Check sheet for the modelled part. Datum: model origin and axes. Units: mm. Face numbers are marked on the shaded views. A direction names the side the tool comes from. Round coordinates to 2 decimals unless told otherwise and drop trailing zeros. Write each loop counter-clockwise with the first axis right and the second up, starting at its lowest first coordinate (ties: lowest second). Pieces come first, ordered by that corner, then holes. Notation, with made-up numbers: M 41,33 L 93,33 A19 cw 93,49 Z; hole C 31,83 d2. An arc over 180 degrees is marked long. Answer in a Markdown table with one row per item.
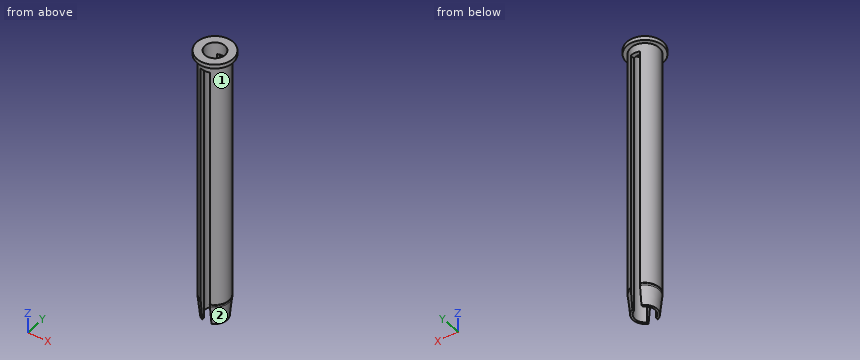
```python
from build123d import *

# Parameters (mm, degrees)
CHAFL_N2_SIZE           = 10
CHAFL_N2_SIZE2          = 1
REDONDEO1_R             = 10
SALIENTE_EXTRUIR1_START = -10.5
CROQUIS3_R              = 7.05
CROQUIS3_R_2            = 6.95
SALIENTE_EXTRUIR1_DEPTH = 0.2
CROQUIS2_W              = 4.5
CROQUIS2_H              = 17.325126262
CORTAR_EXTRUIR1_DEPTH   = 131
CHAFL_N3_SIZE           = 0.1
REDONDEO2_R             = 0.05


# Some blends are built 0.0001 mm under size
with BuildPart() as part:
    # Croquis1 → Revolución1 (revolve)
    with BuildSketch(Plane.YZ, mode=Mode.PRIVATE) as revoluci_n1_sk:
        Polygon((4.95, -68.5), (4.95, 68.5), (8.95, 68.5), (8.95, 66.5), (6.95, 66.5), (6.95, -68.5), align=None)
    revolve(revoluci_n1_sk.sketch.rotate(Axis((0, 0, 0), (0, 0, 1)), 90), axis=Axis((0, 0, 0), (0, 0, 1)))

    # Chaflán2
    chafl_n2_edges = [part.edges().sort_by_distance(p)[0] for p in [
        (6.95, 0, -68.5),
    ]]
    chafl_n2_side = [part.faces().sort_by_distance(p)[0] for p in [
        (6.95, 0, -1),
    ]]
    chamfer(chafl_n2_edges, length=CHAFL_N2_SIZE, length2=CHAFL_N2_SIZE2, reference=chafl_n2_side[0])

    # Redondeo1
    # the kernel refuses this fillet: 10 mm, written as the material it takes off along each edge
    with BuildSketch(Plane(origin=(0, 0, -58.5), x_dir=(-1, 0, 0), z_dir=(0, 1, 0))) as redondeo1_piece_1:
        with BuildLine():
            CenterArc((6.95 - REDONDEO1_R, REDONDEO1_R * 0.0498756211209), REDONDEO1_R, 354.289406863, 5.710593137)
            Line((6.95 - REDONDEO1_R * 0.00496280979001, -REDONDEO1_R * 0.0496280979001), (6.95, 0))
            Line((6.95, 0), (6.95, REDONDEO1_R * 0.0498756211209))
        make_face()
    revolve(axis=Axis((0, 0, -58.5), (0, 0, 1)), mode=Mode.SUBTRACT)

    # Croquis3 → Saliente-Extruir1 (add)
    with BuildSketch(Plane(origin=(0, 0, -68.5), x_dir=(1, 0, 0), z_dir=(0, 0, -1)).offset(SALIENTE_EXTRUIR1_START)):
        with Locations(Location((0, 0, 0), (0, 0, 180))):
            Circle(CROQUIS3_R)
        with Locations(Location((0, 0, 0), (0, 0, 180))):
            Circle(CROQUIS3_R_2, mode=Mode.SUBTRACT)
    extrude(amount=-SALIENTE_EXTRUIR1_DEPTH)

    # Croquis2 → Cortar-Extruir1 (cut)
    with BuildSketch(Plane(origin=(0, 0, -68.5), x_dir=(1, 0, 0), z_dir=(0, 0, -1))):
        Rectangle(CROQUIS2_W, CROQUIS2_H)
    extrude(amount=-CORTAR_EXTRUIR1_DEPTH, mode=Mode.SUBTRACT)

    # Chaflán3
    chafl_n3_edges = [part.edges().sort_by_distance(p)[0] for p in [
        (7.05, 0, -58),
        (-7.05, 0, -58),
    ]]
    chamfer(chafl_n3_edges, length=CHAFL_N3_SIZE - 0.0001)  # a hair under: the kernel refuses the full size

    # Redondeo2
    redondeo2_edges = [part.edges().sort_by_distance(p)[0] for p in [
        (7.05, 0, -57.8),
        (7.05, 0, -57.9001),
        (-7.05, 0, -57.9001),
        (-7.05, 0, -57.8),
    ]]
    fillet(redondeo2_edges, radius=REDONDEO2_R)


solid = part.part
```
1. Section check B-B, the plane x = 0. Record the cut outline in (y, z).
Found:
| item | result |
|---|---|
| outline | M -8.95,66.5 L -6.95,66.5 L -6.95,62.5 L -4.95,62.5 L -4.95,68.5 L -8.95,68.5 Z; M 4.95,62.5 L 6.95,62.5 L 6.95,66.5 L 8.95,66.5 L 8.95,68.5 L 4.95,68.5 Z |
2. Access from +Z, -Z, +X, -X, +Y, -Y to the whole of each face (thin tool, end or side, straight path). Record for the marked faces 1 and 2.
Found:
| item | result |
|---|---|
| face 1 | none |
| face 2 | -Z, +X |
3. Go/stop test with flat-tipped pins: pin 1 (2.5 mm diameter, centred on y = 5, z = 26.5, fed in from -X); pin 2 (1.1 mm diameter, centred on y = -5, z = 29.5, fed in from -X); pin 3 (8 mm diameter, centred on x = 4, z = 11.5, fed in from +Y). Record where each tip stops, or that it passes through.
Found:
| item | result |
|---|---|
| pin 1 | stops at x = -5.85 |
| pin 2 | stops at x = -5.34 |
| pin 3 | stops at y = 6.58 |
4. Section check A-A, the plane z = 8. Record the cut outline in (x, y).
Found:
| item | result |
|---|---|
| outline | M -2.25,-6.58 L -2.25,-4.41 A4.95 cw -2.25,4.41 L -2.25,6.58 A6.95 ccw Z; M 2.25,-6.58 A6.95 ccw 2.25,6.58 L 2.25,4.41 A4.95 cw 2.25,-4.41 Z |
5. Scan lines: L1, parallel to Z at x = -7, y = 4.75; L2, parallel to X at y = -2, z = 44; L3, parallel to Y at x = -4, z = -55. Record each from-to range of solid material in increasing order.
Found:
| item | result |
|---|---|
| L1 | z = 66.5 to 68.5 |
| L2 | x = -6.66 to -4.53, 4.53 to 6.66 |
| L3 | y = -5.68 to -2.92, 2.92 to 5.68 |
